Read the model definition and answer for the solid it produces. Units are mm, in the model's axes. A direction names the side the tool comes from. Give positions to 0.01 mm unless a question says otherwise; leave off trailing zeros. Loops run counter-clockwise (first coordinate to the right, second up) from the corner with the lowest first, then second, coordinate; pieces in that order, holes last. Notation, with made-up numbers: (65.25, 49) - (101.25, 49) arc R33 cw to (101.25, 83) - close; hole circle Ø3 at (35, 23.5). An arc over 180 degrees is marked (long way). Use a Markdown table: item, result. Add a question column.
Item 1: A cutting plane is placed at A-A (x = -10). Determine the outline of the cut face in (y, z).
Item 2: Consider probe 1 along Y at (x, z) = (0, 0.35); probe 2 along Y at (x, z) = (-10, 0.55); probe 3 along X at (y, z) = (-1, 0.65). Determine where each line is inside the solid, lowest interval first. Write a range as [from, to].
Item 3: A cutting plane is placed at B-B (z = -1.6). Determine the outline of the cut face in (x, y), plus the area to 3 significant figures.
Item 4: Which of the six approach directions +Z, -Z, +X, -X, +Y, -Y give full straight-line access (tool end or side, diameter ignored) to faces 5 (the face through (19, 0, -2.5)), 6 (the face through (5, -0.1, 0.5))?
Item 5: For a pull along Y with two mould halves and no side action, classify faces 1 (the face through (0, -4, 1.5)), 2 (the face through (14.77, 11.5, 0.74)), 3 (the face through (-16.9, -16.9, -1.2)), 4 (the face through (-18.5, 0, -1)) as +Y half, -Y half, draft (parallel to the pull), parting line (faces both ways), or undercut.
Item 6: A cutting plane is placed at C-C (y = 0). Determine the outline of the cut face in (x, z), plus the area to 3 significant figures.
Item 7: Each of these flat-tipped pins is pushed along its axis until it touches: P1, Ø12, axis at x = 1.5, y = -11, coming from the -Z side; P2, Ø1.2, axis at x = 5, z = -1.5, coming from the +Y side; P3, Ø6.5, axis at x = 9.5, y = 0, coming from the -Z side; P4, Ø13, axis at x = -10, y = -10, coming from the +Z side. Where does it stop, or does it pass through?
Item 8: A cutting plane is placed at D-D (y = 7). Determine the outline of the cut face in (x, z), plus the area to 3 significant figures.
from build123d import *

# Parameters (mm, degrees)
SKETCH_R        = 5
SKETCH_R_2      = 1.5
PAD_DEPTH       = 1.5
CHAMFER_SIZE2   = 1.25
CHAMFER_SIZE    = 0.65
POCKET_DEPTH    = 1
PAD001_DEPTH    = 2.5
POCKET001_DEPTH = 2.5


with BuildPart() as part:
    # Sketch → Pad (new body)
    with BuildSketch(Plane.XY):
        with BuildLine():
            ThreePointArc((10.665365, -21.5), (24, 0), (10.665365, 21.5))
            Line((-10.665365, 21.5), (10.665365, 21.5))
            ThreePointArc((-10.665365, 21.5), (-24, 0), (-10.665365, -21.5))
            Line((-10.665365, -21.5), (10.665365, -21.5))
        make_face()
        with Locations((10, -10)):
            Circle(SKETCH_R, mode=Mode.SUBTRACT)
        with Locations((-10, -10)):
            Circle(SKETCH_R, mode=Mode.SUBTRACT)
        with Locations((-10, 10)):
            Circle(SKETCH_R, mode=Mode.SUBTRACT)
        with Locations((10, 10)):
            Circle(SKETCH_R, mode=Mode.SUBTRACT)
        Circle(SKETCH_R_2, mode=Mode.SUBTRACT)
    extrude(amount=PAD_DEPTH)

    # Chamfer
    chamfer_edges = [part.edges().sort_by_distance(p)[0] for p in [
        (-1.5, 0, 1.5),
    ]]
    chamfer_side = part.faces().sort_by_distance((-1.5, 0, 0.75))[0]
    chamfer(chamfer_edges, length=CHAMFER_SIZE, length2=CHAMFER_SIZE2, reference=chamfer_side)

    # Sketch001 (on Face3 of Chamfer) → Pocket (cut)
    with BuildSketch(Plane(origin=(0, 0, 0), x_dir=(1, 0, 0), z_dir=(0, 0, -1))):
        with BuildLine():
            ThreePointArc((4, 14.5), (0, 18.5), (-4, 14.5))
            Line((-4, 14.5), (-4, 12))
            ThreePointArc((-4, 12), (0, 8), (4, 12))
            Line((4, 12), (4, 14.5))
        make_face()
        with BuildLine():
            ThreePointArc((-4, -14.5), (0, -18.5), (4, -14.5))
            Line((4, -12), (4, -14.5))
            ThreePointArc((4, -12), (0, -8), (-4, -12))
            Line((-4, -14.5), (-4, -12))
        make_face()
        with BuildLine():
            ThreePointArc((9, 4), (5, 0), (9, -4))
            Line((9, -4), (11, -4))
            ThreePointArc((11, -4), (15, 0), (11, 4))
            Line((11, 4), (9, 4))
        make_face()
        with BuildLine():
            ThreePointArc((-9, -4), (-5, 0), (-9, 4))
            Line((-11, 4), (-9, 4))
            ThreePointArc((-11, 4), (-15, 0), (-11, -4))
            Line((-9, -4), (-11, -4))
        make_face()
    extrude(amount=-POCKET_DEPTH, mode=Mode.SUBTRACT)

    # Sketch002 (on Face3 of Pocket) → Pad001 (join)
    with BuildSketch(Plane(origin=(0, 0, 0), x_dir=(1, 0, 0), z_dir=(0, 0, -1))):
        with BuildLine():
            Line((-20, 13.084724), (-20, -13.084724))
            ThreePointArc((-20, -13.084724), (-16.899852, -16.899852), (-13.084724, -20))
            Line((-13.084724, -20), (13.084724, -20))
            ThreePointArc((13.084724, -20), (16.899852, -16.899852), (20, -13.084724))
            Line((20, -13.084724), (20, 13.084724))
            ThreePointArc((20, 13.084724), (16.899852, 16.899852), (13.084724, 20))
            Line((13.084724, 20), (-13.084724, 20))
            ThreePointArc((-13.084724, 20), (-16.899852, 16.899852), (-20, 13.084724))
        make_face()
    extrude(amount=PAD001_DEPTH)

    # Sketch003 (on Face26 of Pad001) → Pocket001 (cut)
    with BuildSketch(Plane(origin=(0, 0, -2.5), x_dir=(1, 0, 0), z_dir=(0, 0, -1))):
        with BuildLine():
            Line((-18.5, 12.629727), (-18.5, -12.629727))
            ThreePointArc((-18.5, -12.629727), (-15.839192, -15.839192), (-12.629727, -18.5))
            Line((-12.629727, -18.5), (12.629727, -18.5))
            ThreePointArc((12.629727, -18.5), (15.839192, -15.839192), (18.5, -12.629727))
            Line((18.5, -12.629727), (18.5, 12.629727))
            ThreePointArc((18.5, 12.629727), (15.839192, 15.839192), (12.629727, 18.5))
            Line((12.629727, 18.5), (-12.629727, 18.5))
            ThreePointArc((-12.629727, 18.5), (-15.839192, 15.839192), (-18.5, 12.629727))
        make_face()
    extrude(amount=-POCKET001_DEPTH, mode=Mode.SUBTRACT)


solid = part.part
Geometry says:
| question | item | result |
|---|---|---|
| 1 | outline | (-21.5, 0) - (-20, 0) - (-20, -2.5) - (-18.5, -2.5) - (-18.5, 0) - (-15, 0) - (-15, 1.5) - (-21.5, 1.5) - close; (-5, 0) - (-4, 0) - (-4, 1) - (4, 1) - (4, 0) - (5, 0) - (5, 1.5) - (-5, 1.5) - close; (15, 0) - (18.5, 0) - (18.5, -2.5) - (20, -2.5) - (20, 0) - (21.5, 0) - (21.5, 1.5) - (15, 1.5) - close |
| 2 | probe 1 | [-21.5, -18.5], [-8, -1.5], [1.5, 8], [18.5, 21.5] |
| 2 | probe 2 | [-21.5, -15], [-5, -4], [4, 5], [15, 21.5] |
| 2 | probe 3 | [-23.98, -14.87], [-5.13, -1.12], [1.12, 5.13], [14.87, 23.98] |
| 3 | outline | (-20, -13.08) arc R23.9 ccw to (-13.08, -20) - (13.08, -20) arc R23.9 ccw to (20, -13.08) - (20, 13.08) arc R23.9 ccw to (13.08, 20) - (-13.08, 20) arc R23.9 ccw to (-20, 13.08) - close; hole (-18.5, -12.63) arc R22.4 ccw to (-12.63, -18.5) - (12.63, -18.5) arc R22.4 ccw to (18.5, -12.63) - (18.5, 12.63) arc R22.4 ccw to (12.63, 18.5) - (-12.63, 18.5) arc R22.4 ccw to (-18.5, 12.63) - close |
| 3 | area | 209 mm² |
| 4 | face 5 | -Z, +X, -X, +Y, -Y |
| 4 | face 6 | -Z |
| 5 | face 1 | draft |
| 5 | face 2 | undercut |
| 5 | face 3 | -Y half |
| 5 | face 4 | undercut |
| 6 | outline | (-24, 0) - (-20, 0) - (-20, -2.5) - (-18.5, -2.5) - (-18.5, 0) - (-15, 0) - (-15, 1) - (-5, 1) - (-5, 0) - (-1.5, 0) - (-1.5, 0.85) - (-2.75, 1.5) - (-24, 1.5) - close; (1.5, 0) - (5, 0) - (5, 1) - (15, 1) - (15, 0) - (18.5, 0) - (18.5, -2.5) - (20, -2.5) - (20, 0) - (24, 0) - (24, 1.5) - (2.75, 1.5) - (1.5, 0.85) - close |
| 6 | area | 54.2 mm² |
| 7 | P1 | z = 0 |
| 7 | P2 | y = 20 |
| 7 | P3 | z = 1 |
| 7 | P4 | z = 1.5 |
| 8 | outline | (-22.96, 0) - (-20, 0) - (-20, -2.5) - (-18.5, -2.5) - (-18.5, 0) - (-14, 0) - (-14, 1.5) - (-22.96, 1.5) - close; (-6, 0) - (6, 0) - (6, 1.5) - (-6, 1.5) - close; (14, 0) - (18.5, 0) - (18.5, -2.5) - (20, -2.5) - (20, 0) - (22.96, 0) - (22.96, 1.5) - (14, 1.5) - close |
| 8 | area | 52.4 mm² |
